Geometry check sheet. Reference: the model listing, model coordinates, mm. Face numbers are marked on the shaded views. A direction names the side the tool comes from. Give positions to 0.01 mm unless a question says otherwise; leave off trailing zeros. Loops run counter-clockwise (first coordinate to the right, second up) from the corner with the lowest first, then second, coordinate; pieces in that order, holes last. Notation, with made-up numbers: (-8.5, 53.25) -> (40.5, 53.25) arc R8 ccw to (40.5, 67.25) -> close; hole circle Ø6 at (-0.75, 79.5). An arc over 180 degrees is marked (long way). Write item = value, one per line. Start each with the question number.
```python
from build123d import *

# Parameters (mm, degrees)
SKETCH1_R               = 4.95
SKETCH1_R_2             = 2.2
BOSS_EXTRUDE1_DEPTH     = 4
SKETCH2_W               = 47
SKETCH2_H               = 139.3
BOSS_EXTRUDE2_DEPTH     = 19.5
SKETCH3_W               = 41
SKETCH3_H               = 59.3
CUT_EXTRUDE1_DEPTH      = 16
CUT_EXTRUDE3_START      = -3
SKETCH6_R               = 19.5
CUT_EXTRUDE3_DEPTH      = 76
CUT_EXTRUDE4_DEPTH      = 74
CUT_EXTRUDE6_REACH      = 110.634
CUT_EXTRUDE7_DEPTH      = 130.68327973
CUT_EXTRUDE7_DEPTH_BACK = 130.68327973
SKETCH10_W              = 16
SKETCH10_H              = 4
SKETCH12_W              = 47
SKETCH12_H              = 59.3
CUT_EXTRUDE8_DEPTH      = 130.609039197


with BuildPart() as part:
    # Sketch1 → Boss-Extrude1 (new body)
    # profile 1 of 9: a face of its own
    with BuildSketch(Plane(origin=(0, 0, 0), x_dir=(1, 0, 0), z_dir=(0, 1, 0))):
        with Locations((11.630264395, 23.030922034)):
            Circle(SKETCH1_R)
        with Locations(Location((11.630264395, 23.030922034, 0), (0, 0, 270))):
            Circle(SKETCH1_R_2, mode=Mode.SUBTRACT)
    # profile 2 of 9: a face of its own
    with BuildSketch(Plane(origin=(0, 0, 0), x_dir=(1, 0, 0), z_dir=(0, 1, 0))):
        with BuildLine():
            Line((17.830264395, 18.080922034), (17.830264395, 27.980922034))
            Line((17.830264395, 27.980922034), (11.630264395, 27.980922034))
            ThreePointArc((11.630264395, 27.980922034), (15.130442962, 26.5311006), (16.580264395, 23.030922034))
            ThreePointArc((16.580264395, 23.030922034), (15.130442962, 19.530743467), (11.630264395, 18.080922034))
            Line((11.630264395, 18.080922034), (17.830264395, 18.080922034))
        make_face()
    # profile 3 of 9: a face of its own
    with BuildSketch(Plane(origin=(0, 0, 0), x_dir=(1, 0, 0), z_dir=(0, 1, 0))):
        Polygon((64.830264395, -86.169077966), (64.830264395, 18.080922034), (64.830264395, 27.980922034), (64.830264395, 36.030922034), (17.830264395, 36.030922034), (17.830264395, 27.980922034), (17.830264395, 18.080922034), (17.830264395, -86.169077966), (17.830264395, -96.069077966), (17.830264395, -103.269077966), (64.830264395, -103.269077966), (64.830264395, -96.069077966), align=None)
    # profile 4 of 9: a face of its own
    with BuildSketch(Plane(origin=(0, 0, 0), x_dir=(1, 0, 0), z_dir=(0, 1, 0))):
        with Locations((71.030264395, 23.030922034)):
            Circle(SKETCH1_R)
        with Locations(Location((71.030264395, 23.030922034, 0), (0, 0, 270))):
            Circle(SKETCH1_R_2, mode=Mode.SUBTRACT)
    # profile 5 of 9: a face of its own
    with BuildSketch(Plane(origin=(0, 0, 0), x_dir=(1, 0, 0), z_dir=(0, 1, 0))):
        with BuildLine():
            Line((64.830264395, 18.080922034), (71.030264395, 18.080922034))
            ThreePointArc((71.030264395, 18.080922034), (66.080264395, 23.030922034), (71.030264395, 27.980922034))
            Line((71.030264395, 27.980922034), (64.830264395, 27.980922034))
            Line((64.830264395, 27.980922034), (64.830264395, 18.080922034))
        make_face()
    # profile 6 of 9: a face of its own
    with BuildSketch(Plane(origin=(0, 0, 0), x_dir=(1, 0, 0), z_dir=(0, 1, 0))):
        with BuildLine():
            Line((71.030264395, -86.169077966), (64.830264395, -86.169077966))
            Line((64.830264395, -86.169077966), (64.830264395, -96.069077966))
            Line((64.830264395, -96.069077966), (71.030264395, -96.069077966))
            ThreePointArc((71.030264395, -96.069077966), (66.080264395, -91.119077966), (71.030264395, -86.169077966))
        make_face()
    # profile 7 of 9: a face of its own
    with BuildSketch(Plane(origin=(0, 0, 0), x_dir=(1, 0, 0), z_dir=(0, 1, 0))):
        with Locations((71.030264395, -91.119077966)):
            Circle(SKETCH1_R)
        with Locations(Location((71.030264395, -91.119077966, 0), (0, 0, 270))):
            Circle(SKETCH1_R_2, mode=Mode.SUBTRACT)
    # profile 8 of 9: a face of its own
    with BuildSketch(Plane(origin=(0, 0, 0), x_dir=(1, 0, 0), z_dir=(0, 1, 0))):
        with BuildLine():
            Line((11.630264395, -96.069077966), (17.830264395, -96.069077966))
            Line((17.830264395, -96.069077966), (17.830264395, -86.169077966))
            Line((17.830264395, -86.169077966), (11.630264395, -86.169077966))
            ThreePointArc((11.630264395, -86.169077966), (15.130442962, -87.6188994), (16.580264395, -91.119077966))
            ThreePointArc((16.580264395, -91.119077966), (15.130442962, -94.619256533), (11.630264395, -96.069077966))
        make_face()
    # profile 9 of 9: a face of its own
    with BuildSketch(Plane(origin=(0, 0, 0), x_dir=(1, 0, 0), z_dir=(0, 1, 0))):
        with Locations((11.630264395, -91.119077966)):
            Circle(SKETCH1_R)
        with Locations(Location((11.630264395, -91.119077966, 0), (0, 0, 270))):
            Circle(SKETCH1_R_2, mode=Mode.SUBTRACT)
    extrude(amount=BOSS_EXTRUDE1_DEPTH)

    # Sketch2 → Boss-Extrude2 (add)
    with BuildSketch(Plane(origin=(0, 4, 0), x_dir=(1, 0, 0), z_dir=(0, 1, 0))):
        with Locations((41.330264395, -33.619077966)):
            Rectangle(SKETCH2_W, SKETCH2_H)
    extrude(amount=BOSS_EXTRUDE2_DEPTH)

    # Sketch3 → Cut-Extrude1 (cut)
    with BuildSketch(Plane.XZ):
        with Locations((41.330264395, 70.619077966)):
            Rectangle(SKETCH3_W, SKETCH3_H)
    extrude(amount=-CUT_EXTRUDE1_DEPTH, mode=Mode.SUBTRACT)

    # Sketch6 → Cut-Extrude3 (cut)
    with BuildSketch(Plane(origin=(0, 0, -36.030922034), x_dir=(-1, 0, 0), z_dir=(0, 0, -1)).offset(CUT_EXTRUDE3_START)):
        with Locations((-41.330264395, 1)):
            Circle(SKETCH6_R)
    extrude(amount=-CUT_EXTRUDE3_DEPTH, mode=Mode.SUBTRACT)

    # Sketch7 → Cut-Extrude4 (cut)
    with BuildSketch(Plane(origin=(0, 0, -36.030922034), x_dir=(-1, 0, 0), z_dir=(0, 0, -1))):
        with BuildLine():
            Line((-64.830264395, 23.5), (-64.830264395, 4))
            Line((-64.830264395, 4), (-63.629367516, 4))
            ThreePointArc((-63.629367516, 4), (-56.141577638, 17.937384686), (-41.330264395, 23.5))
            Line((-41.330264395, 23.5), (-64.830264395, 23.5))
        make_face()
        with BuildLine():
            Line((-17.830264395, 23.5), (-41.330264395, 23.5))
            ThreePointArc((-41.330264395, 23.5), (-26.518951151, 17.937384686), (-19.031161274, 4))
            Line((-19.031161274, 4), (-17.830264395, 4))
            Line((-17.830264395, 4), (-17.830264395, 23.5))
        make_face()
    extrude(amount=-CUT_EXTRUDE4_DEPTH, mode=Mode.SUBTRACT)

    # Sketch9 → Cut-Extrude6 (cut, up to next)
    with BuildSketch(Plane(origin=(0, 0, 37.969077966), x_dir=(-1, 0, 0), z_dir=(0, 0, -1)), mode=Mode.PRIVATE) as cut_extrude6_sk1:
        with BuildLine():
            Line((-64.830264395, 19), (-54.830264395, 19))
            ThreePointArc((-54.830264395, 19), (-48.44538913, 22.345374206), (-41.330264395, 23.5))
            Line((-41.330264395, 23.5), (-64.830264395, 23.5))
            Line((-64.830264395, 23.5), (-64.830264395, 19))
        make_face()
    cut_extrude6_tool1 = extrude(cut_extrude6_sk1.sketch, amount=-CUT_EXTRUDE6_REACH, mode=Mode.PRIVATE) & part.part
    # Sketch9 → Cut-Extrude6 (cut, up to next)
    with BuildSketch(Plane(origin=(0, 0, 37.969077966), x_dir=(-1, 0, 0), z_dir=(0, 0, -1)), mode=Mode.PRIVATE) as cut_extrude6_sk2:
        with BuildLine():
            Line((-27.830264395, 19), (-17.830264395, 19))
            Line((-17.830264395, 19), (-17.830264395, 23.5))
            Line((-17.830264395, 23.5), (-41.330264395, 23.5))
            ThreePointArc((-41.330264395, 23.5), (-34.215139659, 22.345374206), (-27.830264395, 19))
        make_face()
    cut_extrude6_tool2 = extrude(cut_extrude6_sk2.sketch, amount=-CUT_EXTRUDE6_REACH, mode=Mode.PRIVATE) & part.part
    add(cut_extrude6_tool1.solids().sort_by_distance((57.332082, 21.52882, 37.969078))[0], mode=Mode.SUBTRACT)
    add(cut_extrude6_tool2.solids().sort_by_distance((25.328447, 21.52882, 37.969078))[0], mode=Mode.SUBTRACT)

    # Sketch10 → Cut-Extrude7 (cut, two sides: drawn at the far end of the back side and taken through both)
    with BuildSketch(Plane(origin=(0, 4, 0), x_dir=(1, 0, 0), z_dir=(0, 1, 0)).offset(-CUT_EXTRUDE7_DEPTH_BACK)):
        with Locations((41.330264395, 21.030922034)):
            Rectangle(SKETCH10_W, SKETCH10_H)
    extrude(amount=CUT_EXTRUDE7_DEPTH + CUT_EXTRUDE7_DEPTH_BACK, mode=Mode.SUBTRACT)

    # Sketch12 → Cut-Extrude8 (cut, through all)
    with BuildSketch(Plane(origin=(0, 19, 0), x_dir=(1, 0, 0), z_dir=(0, 1, 0))):
        with Locations((41.330264395, -73.619077966)):
            Rectangle(SKETCH12_W, SKETCH12_H)
    extrude(amount=CUT_EXTRUDE8_DEPTH, mode=Mode.SUBTRACT)


solid = part.part
```
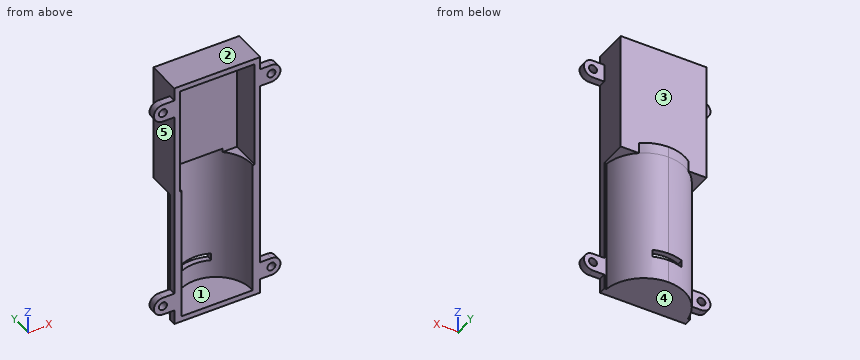
1) Tool access check on the marked faces 1 and 2. Record the directions out of +Z, -Z, +X, -X, +Y, -Y that give a thin tool (end or side, any length) a straight path to the whole face; none if there is none.
2) Depth check by flat-ended pin: pin 1 Ø2 at (y, z) = (5, 40.5) entering from -X; pin 2 Ø1.2 at (x, y) = (15, 2.5) entering from -Z; pin 3 Ø5 at (y, z) = (5, 59.5) entering from +X. Enter the tip coordinate at first touch or a pass-through.
3) Section check B-B (y = 9.5). Enter the section's corners in (x, z), plus the area to 3 significant figures.
4) Thickness scan on line 1 (Z direction, x = 52, y = 5.25); line 2 (X direction, y = 7.25, z = 45); line 3 (Y direction, x = 28.5, z = 53.5). Record the ranges inside material, lowest first.
5) Draft check along Z on the marked faces 3, 4 and 5. Enter one of: released by +Z, released by -Z, zero draft, split by the parting line, or undercut.
6) Section check A-A (z = 66). Enter the section's corners in (x, y).
Check result:
q1.face_1 = -Y
q1.face_2 = +Z, +X, -X, +Y, -Y
q2.pin_1 = 17.83
q2.pin_2 = -27.98
q2.pin_3 = 64.83
q3.outline = (17.83, 37.97) -> (20.5, 37.97) -> (20.5, -36.03) -> (62.16, -36.03) -> (62.16, 37.97) -> (64.83, 37.97) -> (64.83, 103.27) -> (17.83, 103.27) -> close; hole (20.83, 40.97) -> (23.78, 40.97) -> (23.78, -33.03) -> (58.88, -33.03) -> (58.88, 40.97) -> (61.83, 40.97) -> (61.83, 100.27) -> (20.83, 100.27) -> close
q3.area = 1,120 mm2
q4.line_1 = -36.03 to -33.03, 100.27 to 103.27
q4.line_2 = 17.83 to 20.83, 61.83 to 64.83
q4.line_3 = 16 to 19
q5.face_3 = zero draft
q5.face_4 = released by -Z
q5.face_5 = undercut
q6.outline = (17.83, 0) -> (20.83, 0) -> (20.83, 16) -> (61.83, 16) -> (61.83, 0) -> (64.83, 0) -> (64.83, 19) -> (17.83, 19) -> close
